Could you check a few things on this model? Use its own coordinates, in mm. Coordinates: 2 decimals unless noted, no trailing zeros. Order: outer loops, then holes, each group sorted by start corner. A loop starts at its lowest first (then second) coordinate and runs counter-clockwise, first axis right, second up. Notation, with made-up numbers: M -17.75,-9 L -8.75,-9 A24 ccw -8.75,18 Z; hole C 82.25,70 d3. An arc over 180 degrees is marked long. Put each result on its own line as item: value. Start each with the question number.
```python
from build123d import *

# Parameters (mm, degrees)
F0_R     = 16.0774395659
F1_DEPTH = 5
F2_SIZE  = 1
F5_SIZE  = 1


# Not quite as in the source:
# - the program builds the solid bodies; features that only make, move or delete a surface that nothing else refers to are left out


with BuildPart() as f1:
    # F0 (on Top) → F1 (new body)
    with BuildSketch(Plane.XY):
        Circle(F0_R)
    extrude(amount=F1_DEPTH)

    # F2
    f2_edges = [f1.edges().sort_by_distance(p)[0] for p in [
        (-16.07744, 0, 5),
    ]]
    chamfer(f2_edges, length=F2_SIZE)

    # F5
    f5_edges = [f1.edges().sort_by_distance(p)[0] for p in [
        (-16.07744, 0, 0),
    ]]
    chamfer(f5_edges, length=F5_SIZE)


solid = f1.part
```
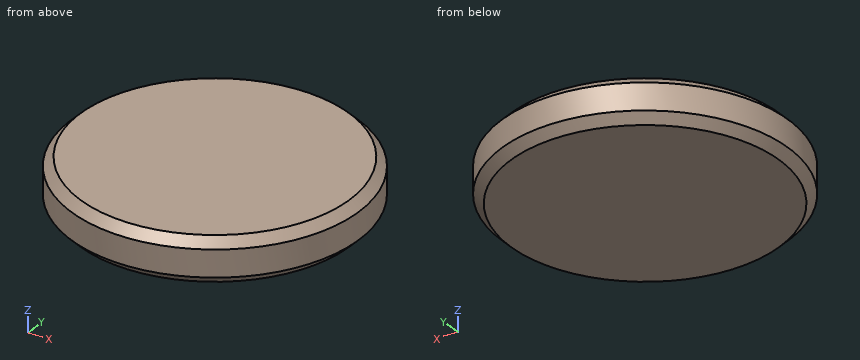
Item 1: For pin 1 Ø1.5 at (x, y) = (-10, -12.5) entering from +Z; pin 2 Ø2 at (x, z) = (-11.5, 1) entering from +Y; pin 3 Ø1.5 at (x, z) = (-7, 3.5) entering from +Y, each with a flat end and sliding along its axis, tell me the tip position at first contact or that it passes through.
Item 2: I need wall thicknesses on probe 1 along Y at (x, z) = (0, 3.95); probe 2 along Y at (x, z) = (-2, 0.65); probe 3 along X at (y, z) = (-13, 4.2). Which ranges of each line are inside material? Lowest first, please.
Item 3: If we section it at A-A on z = 2.15: Write out the boundary of the cut face in (x, y).
Geometry check:
1. pin 1: stops at z = 4.82
1. pin 2: stops at y = 12.18
1. pin 3: stops at y = 14.81
2. probe 1: y = -16.08 to 16.08
2. probe 2: y = -15.6 to 15.6
2. probe 3: x = -9.12 to 9.12
3. outline: C 0,0 d32.15
